Part model, mm, in its own coordinate system. A direction names the side the tool comes from. Give positions to 0.01 mm unless a question says otherwise; leave off trailing zeros. Order: outer loops, then holes, each group sorted by start corner. A loop starts at its lowest first (then second) coordinate and runs counter-clockwise, first axis right, second up.
from build123d import *

# Parameters (mm, degrees)
F0_R     = 10.16
F1_DEPTH = 6.35


with BuildPart() as f1:
    # F0 (on Top) → F1 (new body)
    with BuildSketch(Plane.XY):
        with BuildLine():
            ThreePointArc((25.123501, -0.053256), (13.106305, 7.566929), (12.515629, 21.784218))
            ThreePointArc((12.515629, 21.784218), (13.106305, 22.913071), (13.788583, 23.989038))
            ThreePointArc((13.788583, 23.989038), (0, 45.72), (-13.788583, 23.989038))
            ThreePointArc((-13.788583, 23.989038), (-13.106305, 22.913071), (-12.515629, 21.784218))
            ThreePointArc((-12.515629, 21.784218), (-11.063539, 14.602974), (-13.106305, 7.566929))
            ThreePointArc((-13.106305, 7.566929), (-18.178316, 2.279819), (-25.123501, -0.053256))
            ThreePointArc((-25.123501, -0.053256), (-26.396454, -0.106143), (-27.669408, -0.053256))
            ThreePointArc((-27.669408, -0.053256), (-39.594681, -22.86), (-13.880825, -23.935782))
            ThreePointArc((-13.880825, -23.935782), (-13.290149, -22.806929), (-12.607872, -21.730962))
            ThreePointArc((-12.607872, -21.730962), (0, -15.133857), (12.607872, -21.730962))
            ThreePointArc((12.607872, -21.730962), (13.290149, -22.806929), (13.880825, -23.935782))
            ThreePointArc((13.880825, -23.935782), (39.594681, -22.86), (27.669408, -0.053256))
            ThreePointArc((27.669408, -0.053256), (26.396454, -0.106143), (25.123501, -0.053256))
        make_face()
        with Locations((-26.396454, -15.24)):
            Circle(F0_R, mode=Mode.SUBTRACT)
        with Locations((26.396454, -15.24)):
            Circle(F0_R, mode=Mode.SUBTRACT)
        Circle(F0_R, mode=Mode.SUBTRACT)
        with Locations((0, 30.48)):
            Circle(F0_R, mode=Mode.SUBTRACT)
    extrude(amount=F1_DEPTH)


solid = f1.part
Item 1: Band-saw the part on C-C on z = 4. List the corners of the cut face in (x, y).
Item 2: Which spindle directions (+Z, -Z, +X, -X, +Y, -Y) get a long thin tool onto all of the face, cutting with end or side? Do faces 1 (the face through (13.28, -22.79, 3.13)), 2 (the face through (26.414, -0.106, 3.131)), 3 (the face through (13.1, 22.9, 3.1)). Say none if no direction does.
Item 3: Drop flat-ended pins along their axis: P1, Ø12, axis at x = 0, y = 30.48, coming from the +Z side; P2, Ø2, axis at y = 3, z = 5, coming from the +X side; P3, Ø1.5, axis at y = 37, z = 4, coming from the -X side. Give the stop position or say it passes through.
Item 4: Drill centre lines: probe 1 along Y at (x, z) = (0.5, 2.25); probe 2 along Y at (x, z) = (0, 3); probe 3 along X at (y, z) = (-15, 3.75). Where is each one in solid material? Low to high.
Item 5: Band-saw the part on A-A on x = 0. List the corners of the cut face in (y, z).
Item 6: Pull direction X, two halves, no side cores. Call faces 4 (the face through (-13.1, 22.9, 3.1)), 5 (the face through (-1.323, 10.074, 3.131)), 6 (the face through (13.21, 7.39, 3.13)): released by +X, released by -X, zero draft, split by the parting line, or undercut.
Item 7: Band-saw the part on B-B on y = 30.48. List the corners of the cut face in (x, z).
Item 8: Band-saw the part on D-D on y = -6. List the corners of the cut face in (x, z).
Working result:
1. outline: (-27.67, -0.05) arc R15.24 ccw (long way) to (-13.88, -23.94) arc R15.35 cw to (-12.61, -21.73) arc R15.35 cw to (12.61, -21.73) arc R15.35 cw to (13.88, -23.94) arc R15.24 ccw (long way) to (27.67, -0.05) arc R15.35 cw to (25.12, -0.05) arc R15.35 cw to (12.52, 21.78) arc R15.35 cw to (13.79, 23.99) arc R15.24 ccw (long way) to (-13.79, 23.99) arc R15.35 cw to (-12.52, 21.78) arc R15.35 cw to (-25.12, -0.05) arc R15.35 cw to start; hole circle Ø20.32 at (-26.4, -15.24); hole circle Ø20.32 at (0, 0); hole circle Ø20.32 at (0, 30.48); hole circle Ø20.32 at (26.4, -15.24)
2. face 1: +Z, -Z, -Y
2. face 2: +Z, -Z, +Y
2. face 3: +Z, -Z, +X
3. P1: passes through
3. P2: stops at x = 18.64
3. P3: stops at x = -14.11
4. probe 1: y = -15.14 to -10.15, 10.15 to 20.33, 40.63 to 45.71
4. probe 2: y = -15.13 to -10.16, 10.16 to 20.32, 40.64 to 45.72
4. probe 3: x = -41.63 to -36.55, -16.24 to 16.24, 36.55 to 41.63
5. outline: (-15.13, 0) - (-10.16, 0) - (-10.16, 6.35) - (-15.13, 6.35) - close; (10.16, 0) - (20.32, 0) - (20.32, 6.35) - (10.16, 6.35) - close; (40.64, 0) - (45.72, 0) - (45.72, 6.35) - (40.64, 6.35) - close
6. face 4: released by -X
6. face 5: undercut
6. face 6: released by +X
7. outline: (-15.24, 0) - (-10.16, 0) - (-10.16, 6.35) - (-15.24, 6.35) - close; (10.16, 0) - (15.24, 0) - (15.24, 6.35) - (10.16, 6.35) - close
8. outline: (-38.52, 0) - (-30.62, 0) - (-30.62, 6.35) - (-38.52, 6.35) - close; (-22.17, 0) - (-8.2, 0) - (-8.2, 6.35) - (-22.17, 6.35) - close; (8.2, 0) - (22.17, 0) - (22.17, 6.35) - (8.2, 6.35) - close; (30.62, 0) - (38.52, 0) - (38.52, 6.35) - (30.62, 6.35) - close
